Autodesk Inventor part; units mm, degrees
ref_plane "YZ Plane" through (0, 0, 0) normal (1, 0, 0) x (0, 1, 0)
ref_plane "XZ Plane" through (0, 0, 0) normal (0, 1, 0) x (-1, 0, 0)
ref_plane "XY Plane" through (0, 0, 0) normal (0, 0, 1) x (1, 0, 0)
sketch "base" plane through (0, 0, 0) normal (0, 1, 0) x (-1, 0, 0)
  line L0 (0, 0) -> (0, -20)
  line L1 (0, -20) -> (10, -20)
  line L2 (10, -20) -> (10, 0)
  line L3 (10, 0) -> (0, 0)
  dimension "d186" = 20
  dimension "d187" = 10
extrude "Extrusión29" add sketch "base" along normal blind 50
sketch "Boceto41" plane through (0, 50, 0) normal (0, 1, 0) x (1, 0, 0)
  line L0 (0, 20) -> (5, 20)
  line L1 (5, 20) -> (5, 0)
  line L2 (-10, 0) -> (0, 0)
  line L3 (5, 0) -> (-10, 0)
  line L4 (-10, 0) -> (-10, 20)
  line L5 (-10, 20) -> (5, 20)
  dimension "d190" = 5
extrude "Extrusión30" add sketch "Boceto41" along normal blind 15
sketch "Boceto42" plane through (-10, 0, 0) normal (0, 0, 1) x (1, 0, 0)
  line L0 (15, 50) -> (10, 50)
  line L1 (15, 50) -> (0, 50)
  line L2 (0, 0) -> (0, 65)
  line L3 (0, 50) -> (0, 65)
  line L4 (0, 65) -> (15, 65)
  line L5 (0, 65) -> (15, 65)
  line L6 (15, 65) -> (15, 50)
  point P0 (10, 0)
extrude "Extrusión31" add sketch "Boceto42" along normal blind 10
sketch "Boceto45" plane through (5, 50, -20) normal (1, 0, 0) x (0, 0, -1)
  line L0 (0, -50) -> (0, 15)
  line L1 (0, 0) -> (0, 15)
  line L2 (0, 7.5) -> (-6, 7.5)
  point P0 (-20, -50)
  dimension "d200" = 6
hole "Agujero1" at (5, 57.5, -14) direction (-1, 0, 0) diameter 3.2 end through all
sketch "Boceto51" plane through (-10, 0, -20) normal (-1, 0, 0) x (0, 0, 1)
  circle A0 centre (6, 57.5) radius 1.6
  circle A1 centre (6, 57.5) radius 1.6
  point P0 (20, 0)
hole "Agujero2" at (-10, 57.5, -14) direction (1, 0, 0) diameter 3.2 depth 30 counterbore diameter 10 counterbore depth 5
sketch "Boceto52" plane through (0, 0, 0) normal (0, -1, 0) x (1, 0, 0)
  line L0 (0, 0) -> (0, -20)
  line L1 (10, 0) -> (10, -20)
  line L2 (-10, 0) -> (0, 0)
  line L3 (-20, 0) -> (-20, -20)
  line L4 (-20, -20) -> (-20, -21)
  line L5 (-20, 0) -> (-20, 1)
  line L6 (10, 0) -> (10, 1)
  line L7 (10, -20) -> (10, -21)
  line L8 (10, -21) -> (-20, -21)
  line L9 (10, 1) -> (-20, 1)
  dimension "d237" = 10
  dimension "d238" = 20
  dimension "d239" = 10
  dimension "d240" = 20
  dimension "d241" = 1
  dimension "d242" = 1
  dimension "d244" = 1
extrude "Extrusión36" add sketch "Boceto52" against normal blind 3
sketch "Boceto53" plane through (0, 3, 0) normal (0, 1, 0) x (1, 0, 0)
  line L0 (-20, 21) -> (-20, -1)
  line L1 (-19, 0) -> (-19, 20)
  line L2 (-19, 20) -> (9, 20)
  line L3 (9, 20) -> (9, 0)
  line L4 (9, 0) -> (-19, 0)
  line L5 (-20, 21) -> (-20, -1)
  line L6 (10, -1) -> (10, 21)
  line L7 (-20, -1) -> (10, -1)
  line L8 (10, -1) -> (10, 21)
  line L9 (10, 21) -> (-20, 21)
  line L10 (-20, 21) -> (-20, -1)
  point P0 (0, 0)
  dimension "d248" = 20
  dimension "d249" = 28
  dimension "d250" = 20
extrude "Extrusión37" add sketch "Boceto53" along normal blind 1
sketch "Boceto54" plane through (0, 3, 0) normal (0, 1, 0) x (1, 0, 0)
  circle A0 centre (-14, 10) radius 1.7
  circle A1 centre (4, 10) radius 1.7
  dimension "d259" = 3.4
  dimension "d261" = 3.4
extrude "Extrusión38" cut sketch "Boceto54" against normal blind 39
sketch "Boceto55" plane through (5, 50, -20) normal (1, 0, 0) x (0, 0, -1)
  line L0 (-30, 15) -> (-30, 0)
  line L1 (0, 15) -> (-30, 15)
  line L2 (-30, 15) -> (-30, 0)
  line L3 (-30, 0) -> (0, 0)
  line L4 (0, 0) -> (0, 15)
  circle A0 centre (-6, 7.5) radius 1.6
  circle A1 centre (-6, 7.5) radius 2.1
  point P0 (-20, -50)
  dimension "d264" = 4.2
extrude "Extrusión39" cut sketch "Boceto55" against normal blind 0.5 contours L1 L4 L3 L0
properties part number "detector curvament fil"
Geometry: final body of the model. Coordinates: model frame, mm. A direction names the side the tool comes from. Give positions to 0.01 mm unless a question says otherwise; leave off trailing zeros. Write each loop counter-clockwise with the first axis right and the second up, starting at its lowest first coordinate (ties: lowest second). Pieces come first, ordered by that corner, then holes.
1. Section query D-D, the plane z = -10. Return loops of the section in (x, y).
2. Line query: probe 1 along Y at (x, z) = (0.25, -14); probe 2 along Y at (x, z) = (2.75, -3.5); probe 3 along Z at (x, y) = (4, 2.25). Output: solid intervals per line, ascending.
3. Pin query (flat end, axial travel): P1, Ø1.1, axis at x = -14, y = 3.5, coming from the +Z side; P2, Ø4.5, axis at y = 58, z = -13, coming from the +X side; P3, Ø1.5, axis at x = -0.5, z = 3, coming from the -Y side; P4, Ø3, axis at y = 57.5, z = -14, coming from the -X side. Return the tip coordinate at first contact, or that it passes through.
4. Section query C-C, the plane x = -7.5. Return loops of the section in (y, z).
5. Reachability of faces 1 (the flat face through (-5, 56, -15)), 2 (the flat face through (6, 3, -10)), 3 (the flat face through (5, 59, -13)) from +Z, -Z, +X, -X, +Y, -Y: full face, straight path, thin tool, end or side. Return the list, or none.
6. Section query A-A, the plane z = -14. Return loops of the section in (x, y), then the cut area to 3 significant figures.
7. Draft query along Y for faces 4 (the flat face through (-3, 65, -5)), 5 (the flat face through (-5, 27, 0)), 6 (the cylindrical face through (5.57, 1.52, -9.35)), 7 (the flat face through (-5, 0, -10)). Return one class per face: released by +Y, released by -Y, zero draft, split by the parting line, or undercut.
8. Section query B-B, the plane y = 57.5. Return loops of the section in (x, z), then the cut area to 3 significant figures.
Computed:
1. outline: (-20, 0) - (-15.7, 0) - (-15.7, 3) - (-19, 3) - (-19, 4) - (-20, 4) - close; (-12.3, 0) - (2.3, 0) - (2.3, 3) - (0, 3) - (0, 50) - (4.5, 50) - (4.5, 65) - (-10, 65) - (-10, 60.5) - (-5, 60.5) - (-5, 54.5) - (-10, 54.5) - (-10, 3) - (-12.3, 3) - close; (5.7, 0) - (10, 0) - (10, 4) - (9, 4) - (9, 3) - (5.7, 3) - close
2. probe 1: y = 0 to 3, 50 to 55.9, 59.1 to 65
2. probe 2: y = 0 to 3, 50 to 65
2. probe 3: z = -21 to -11.7, -8.3 to 1
3. P1: stops at z = 1
3. P2: stops at x = 5
3. P3: stops at y = 50
3. P4: passes through
4. outline: (0, -21) - (4, -21) - (4, -20) - (65, -20) - (65, 10) - (50, 10) - (50, 0) - (4, 0) - (4, 1) - (0, 1) - close; hole circle Ø10 at (57.5, -14)
5. face 1: -X
5. face 2: none
5. face 3: +Z, -Z, +X, +Y
6. outline: (-20, 0) - (10, 0) - (10, 4) - (9, 4) - (9, 3) - (0, 3) - (0, 50) - (4.5, 50) - (4.5, 55.4) - (5, 55.4) - (5, 55.9) - (-5, 55.9) - (-5, 52.5) - (-10, 52.5) - (-10, 3) - (-19, 3) - (-19, 4) - (-20, 4) - close; (-10, 62.5) - (-5, 62.5) - (-5, 59.1) - (5, 59.1) - (5, 59.6) - (4.5, 59.6) - (4.5, 65) - (-10, 65) - close
6. area: 700 mm2
7. face 4: released by +Y
7. face 5: undercut
7. face 6: zero draft
7. face 7: released by -Y
8. outline: (-10, -20) - (4.5, -20) - (4.5, -16.1) - (5, -16.1) - (5, -15.6) - (-5, -15.6) - (-5, -19) - (-10, -19) - close; (-10, -9) - (-5, -9) - (-5, -12.4) - (5, -12.4) - (5, -11.9) - (4.5, -11.9) - (4.5, 10) - (-10, 10) - close
8. area: 355 mm2
